```python
from build123d import *

# Parameters (mm, degrees)
WEDGE_GENERAL_SHAPE_DEPTH      = 73
SIDE_FILLET_R                  = 1.5
CORNER_START                   = -3
CORNER_FILLET_DEPTH            = 4
KNIFE_EDGE_REMOVER_R           = 0.125
CARD_GUIDE_SIZE                = 0.5
SKETCH14_W                     = 47
SKETCH14_H                     = 7
BABY_WEDGE_SHORTENER_DEPTH     = 10
BABY_WEDGE_SIDE_FILLET_R       = 1.5
BABY_START                     = -3
BABY_WEDGE_CORNER_FILLET_DEPTH = 4
M2X0_4_TAPPED_HOLE2_D          = 1.6
BABY_BITE_FILLET_R             = 0.25


with BuildPart() as part:
    # Sketch2 → Wedge General Shape (new body)
    with BuildSketch(Plane(origin=(0, 0, 0), x_dir=(0, 0, -1), z_dir=(1, 0, 0))):
        Polygon((0, 7), (0, 0), (2, 3.464101615), (2, 7), align=None)
    extrude(amount=WEDGE_GENERAL_SHAPE_DEPTH)

    # Side Fillet
    side_fillet_edges = [part.edges().sort_by_distance(p)[0] for p in [
        (73, 1.732050808, -1),
        (0, 1.732050808, -1),
    ]]
    fillet(side_fillet_edges, radius=SIDE_FILLET_R)

    # Corner Fillet: read off the stored shape, not the designer's step
    # Corner Fillet outline → Corner Fillet (cut)
    with BuildSketch(Plane.XY.offset(CORNER_START)):
        with BuildLine():
            Line((73, 7), (71, 7))
            ThreePointArc((71, 7), (72.414213562, 6.414213562), (73, 5))
            Line((73, 5), (73, 7))
        make_face()
        with BuildLine():
            ThreePointArc((0, 5), (0.585786438, 6.414213562), (2, 7))
            Line((2, 7), (0, 7))
            Line((0, 7), (0, 5))
        make_face()
    extrude(amount=CORNER_FILLET_DEPTH, mode=Mode.SUBTRACT)

    # Knife Edge Remover
    # the kernel refuses this fillet: 0.125 mm, written as the material it takes off along each edge
    with BuildSketch(Plane(origin=(0.333734123, 0, 0), x_dir=(0, 1, 0), z_dir=(1, 0, 0))) as knife_edge_remover_piece_1:
        with BuildLine():
            CenterArc((KNIFE_EDGE_REMOVER_R * 3.73205080757, -KNIFE_EDGE_REMOVER_R), KNIFE_EDGE_REMOVER_R, 90, 150)
            Line((KNIFE_EDGE_REMOVER_R * 3.23205080757, -KNIFE_EDGE_REMOVER_R * 1.86602540378), (0, 0))
            Line((0, 0), (KNIFE_EDGE_REMOVER_R * 3.73205080757, 0))
        make_face()
    extrude(amount=72.332531755, mode=Mode.SUBTRACT)

    # Card Guide
    # the kernel refuses this chamfer: 0.5 mm, written as the material it takes off along each edge
    with BuildSketch(Plane(origin=(-0.18593054, 7, 0), x_dir=(0, -1, 0), z_dir=(1, 0, 0))) as card_guide_piece_1:
        Polygon((CARD_GUIDE_SIZE, 0), (0, CARD_GUIDE_SIZE), (0, 0), align=None)
    extrude(amount=73.37186108, mode=Mode.SUBTRACT)

    # Sketch14 → Baby Wedge Shortener (cut)
    with BuildSketch(Plane.XY):
        with Locations((23.5, 3.5)):
            Rectangle(SKETCH14_W, SKETCH14_H)
    extrude(amount=-BABY_WEDGE_SHORTENER_DEPTH, mode=Mode.SUBTRACT)

    # Baby Wedge Side Fillet
    # the kernel refuses this fillet: 1.5 mm, written as the material it takes off along each edge
    with BuildSketch(Plane(origin=(47, -2.843588913, 1.641746825), x_dir=(0, 0.49999999999999317, 0.8660254037844426), z_dir=(0, 0.8660254037844427, -0.4999999999999932))) as baby_wedge_side_fillet_piece_1:
        with BuildLine():
            CenterArc((BABY_WEDGE_SIDE_FILLET_R, BABY_WEDGE_SIDE_FILLET_R), BABY_WEDGE_SIDE_FILLET_R, 180, 90)
            Line((0, BABY_WEDGE_SIDE_FILLET_R), (0, 0))
            Line((0, 0), (BABY_WEDGE_SIDE_FILLET_R, 0))
        make_face()
    extrude(amount=11.033493649, mode=Mode.SUBTRACT)

    # Baby Wedge Corner Fillet: read off the stored shape, not the designer's step
    # Baby Wedge Corner Fillet outline → Baby Wedge Corner Fillet (cut)
    with BuildSketch(Plane.XY.offset(BABY_START)):
        with BuildLine():
            ThreePointArc((47, 5), (47.585786438, 6.414213562), (49, 7))
            Line((49, 7), (47, 7))
            Line((47, 7), (47, 5))
        make_face()
    extrude(amount=BABY_WEDGE_CORNER_FILLET_DEPTH, mode=Mode.SUBTRACT)

    # M2x0.4 Tapped Hole2 (through all)
    with Locations(Plane(origin=(0, 0, -2), x_dir=(-1, 0, 0), z_dir=(0, 0, -1))):
        with Locations((-68.5, 3.702003175), (-51.5, 3.702003175)):
            Hole(M2X0_4_TAPPED_HOLE2_D / 2)

    # Baby Bite Fillet
    baby_bite_fillet_edges = [part.edges().sort_by_distance(p)[0] for p in [
        (47.790438534, 6.592784059, -2),
        (72.209561466, 6.592784059, -2),
        (60, 7, -2),
    ]]
    fillet(baby_bite_fillet_edges, radius=BABY_BITE_FILLET_R)


solid = part.part
```
Input: part model. Units: mm. Frame: model coordinates. Give positions to 0.01 mm unless a question says otherwise; leave off trailing zeros. Put each result on its own line as item: value.
Item 1: Draft query along Y for faces 1 (the cylindrical face through (47.57, 6.4, -0.89)), 2 (the cylindrical face through (68.93, 4.377, -0.986)), 3 (the flat face through (59.839, 1.913, -1.104)). Return one class per face: +Y half, -Y half, draft (parallel to the pull), parting line (faces both ways), or undercut.
Found:
face 1: +Y half
face 2: undercut
face 3: -Y half
Item 2: Section query C-C, the plane y = 4.25. Count the separate pieces of the cut face and the enclosed holes in it, then the cut area to 3 significant figures.
Found:
separate pieces: 3
enclosed holes: 0
area: 47.0 mm^2
Item 3: Ray query, L1, parallel to X at y = 4.25, z = -1.55; L2, parallel to X at y = 4, z = -1.9; L3, parallel to Y at x = 51.5, z = -1.1. Return the intervals inside material, ascending. Write a range as from..to.
Found:
L1: x = 47.18..50.92, 52.08..67.92, 69.08..72.82
L2: x = 47.53..50.76, 52.24..67.76, 69.24..72.47
L3: y = 1.91..2.9, 4.5..7
Item 4: Contact query for flat-ended pins moving along their axis: pin 1 (2 mm diameter, centred on x = 56, y = 5, fed in from +Z); pin 2 (1.3 mm diameter, centred on x = 68.5, y = 3.7, fed in from +Z). Output: stop coordinate, or through.
Found:
pin 1: stops at z = 0
pin 2: passes through
